from build123d import *
from OCP.BRepFilletAPI import BRepFilletAPI_MakeChamfer

# Parameters (mm, degrees)
SKETCH_2_W          = 8
SKETCH_2_H          = 200
EXTRUDE_1_DEPTH     = 10
SKETCH_3_W          = 2
SKETCH_3_H          = 30
EXTRUDE_2_DEPTH     = 10
SKETCH_4_R          = 1.65
CUT_EXTRUDE_1_DEPTH = 20
SKETCH_5_W          = 4
SKETCH_5_H          = 100
CUT_EXTRUDE_2_DEPTH = 20
CHAMFER_1_SIZE      = 5
CHAMFER_1_SIZE2     = 13.737387097
SKETCH_6_W          = 2
SKETCH_6_H          = 27.5
EXTRUDE_3_DEPTH     = 15
SKETCH_7_R          = 1.65
CUT_EXTRUDE_3_DEPTH = 10
SKETCH_8_R          = 1.6
CUT_EXTRUDE_4_DEPTH = 10


with BuildPart() as part:
    # 草图2 → 凸台-拉伸1 (new body)
    with BuildSketch(Plane(origin=(0, 0, 0), x_dir=(1, 0, 0), z_dir=(0, 1, 0))):
        Rectangle(SKETCH_2_W, SKETCH_2_H)
    extrude(amount=EXTRUDE_1_DEPTH)

    # 草图3 → 凸台-拉伸2 (add)
    with BuildSketch(Plane(origin=(0, 10, 0), x_dir=(1, 0, 0), z_dir=(0, 1, 0))):
        with Locations((-3, 0)):
            Rectangle(SKETCH_3_W, SKETCH_3_H)
        with Locations((3, 0)):
            Rectangle(SKETCH_3_W, SKETCH_3_H)
    extrude(amount=EXTRUDE_2_DEPTH)

    # 草图4 → 切除-拉伸1 (cut)
    with BuildSketch(Plane.ZY.offset(4)):
        with Locations((-7.5, 15)):
            Circle(SKETCH_4_R)
        with Locations((7.5, 15)):
            Circle(SKETCH_4_R)
    extrude(amount=-CUT_EXTRUDE_1_DEPTH, mode=Mode.SUBTRACT)

    # 草图5 → 切除-拉伸2 (cut)
    with BuildSketch(Plane(origin=(0, 10, 0), x_dir=(1, 0, 0), z_dir=(0, 1, 0))):
        Rectangle(SKETCH_5_W, SKETCH_5_H)
    extrude(amount=-CUT_EXTRUDE_2_DEPTH, mode=Mode.SUBTRACT)

    # 倒角1: one chamfer whose edges measure the first distance from different faces: ONE call of the kernel's chamfer builder (chamfer() names one face for all edges)
    chamfer_1_edges_1 = [part.edges().sort_by_distance(p)[0] for p in [
        (0, 0, 100),
    ]]
    chamfer_1_side_1 = [part.faces().sort_by_distance(p)[0] for p in [
        (0, 5, 100),
    ]]
    chamfer_1_edges_2 = [part.edges().sort_by_distance(p)[0] for p in [
        (0, 0, -100),
    ]]
    chamfer_1_side_2 = [part.faces().sort_by_distance(p)[0] for p in [
        (0, 5, -100),
    ]]
    chamfer_1 = BRepFilletAPI_MakeChamfer(part.part.solid().wrapped)
    for e in chamfer_1_edges_1:
        chamfer_1.Add(CHAMFER_1_SIZE, CHAMFER_1_SIZE2, e.wrapped, chamfer_1_side_1[0].wrapped)  # the first distance lies on this face
    for e in chamfer_1_edges_2:
        chamfer_1.Add(CHAMFER_1_SIZE, CHAMFER_1_SIZE2, e.wrapped, chamfer_1_side_2[0].wrapped)  # the first distance lies on this face
    add(Compound.cast(chamfer_1.Shape()), mode=Mode.REPLACE)

    # 草图6 → 凸台-拉伸3 (add)
    with BuildSketch(Plane(origin=(0, 10, 0), x_dir=(1, 0, 0), z_dir=(0, 1, 0))):
        with Locations((-3, 43.75)):
            Rectangle(SKETCH_6_W, SKETCH_6_H)
    extrude_3 = extrude(amount=EXTRUDE_3_DEPTH)

    # 镜向2: 凸台-拉伸3 across plane
    add(extrude_3.mirror(Plane.XY))

    # 草图7 → 切除-拉伸3 (cut)
    with BuildSketch(Plane.ZY.offset(4)):
        with Locations((80, 5)):
            Circle(SKETCH_7_R)
        with Locations((65, 5)):
            Circle(SKETCH_7_R)
        with Locations((-65, 5)):
            Circle(SKETCH_7_R)
        with Locations((-80, 5)):
            Circle(SKETCH_7_R)
    extrude(amount=-CUT_EXTRUDE_3_DEPTH, mode=Mode.SUBTRACT)

    # 草图8 → 切除-拉伸4 (cut)
    with BuildSketch(Plane(origin=(-2, 0, 0), x_dir=(0, 0, -1), z_dir=(1, 0, 0))):
        with Locations((-52.235249282, 21.351499314)):
            Circle(SKETCH_8_R)
        with Locations((-38.268733006, 15.880080566)):
            Circle(SKETCH_8_R)
        with Locations((38.268733006, 15.880080566)):
            Circle(SKETCH_8_R)
        with Locations((52.235249282, 21.351499314)):
            Circle(SKETCH_8_R)
    extrude(amount=-CUT_EXTRUDE_4_DEPTH, mode=Mode.SUBTRACT)


solid = part.part
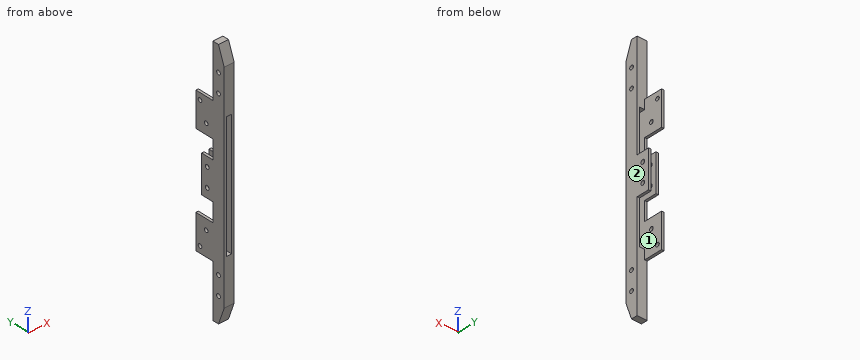
Verification items for the finished model (mm, model axes). Face numbers are marked on the shaded views. Give positions to 0.01 mm unless a question says otherwise; leave off trailing zeros. Write each loop counter-clockwise with the first axis right and the second up, starting at its lowest first coordinate (ties: lowest second). Pieces come first, ordered by that corner, then holes. Notation, with made-up numbers: (24.25, 1) -> (81.25, 1) arc R26 ccw to (81.25, 38) -> close; hole circle Ø10 at (2.25, 15.5). An arc over 180 degrees is marked (long way). Use CSV: the item, a comma, the result in double quotes.
(1) Release check for a two-part mould opening along Z. For the marked faces 1 and 2 record: +Z half, -Z half, draft (parallel to the pull), parting line (faces both ways), or undercut.
Derived:
face 1,"undercut"
face 2,"draft"
(2) Sectioned sample at C-C (z = 69.5). Record the cut outline in (x, y).
Derived:
outline,"(-4, 0) -> (4, 0) -> (4, 10) -> (-4, 10) -> close"
(3) Sectioned sample at B-B (z = -65). Record the cut outline in (x, y).
Derived:
outline,"(-4, 0) -> (4, 0) -> (4, 3.35) -> (-4, 3.35) -> close; (-4, 6.65) -> (4, 6.65) -> (4, 10) -> (-4, 10) -> close"
(4) Material ranges on L1, parallel to Z at x = -3.25, y = 11; L2, parallel to X at y = 15.25, z = 11.5; L3, parallel to Z at x = 1.5, y = 7.5, recorded low to high.
Derived:
L1,"z = -57.5 to -30, -15 to 15, 30 to 57.5"
L2,"x = -4 to -2, 2 to 4"
L3,"z = -100 to -50, 50 to 100"
(5) Go/stop test with flat-tipped pins: pin 1 (2.5 mm diameter, centred on y = 15, z = -7.5, fed in from +X); pin 2 (3.5 mm diameter, centred on y = 15.88, z = 38.27, fed in from +X); pin 3 (1 mm diameter, centred on x = -3, y = 21, fed in from -Z); pin 4 (2 mm diameter, centred on x = -3, y = 13.5, fed in from +Z). Record where each tip stops, or that it passes through.
Derived:
pin 1,"passes through"
pin 2,"stops at x = -2"
pin 3,"stops at z = -57.5"
pin 4,"stops at z = 57.5"
(6) Sectioned sample at A-A (z = 1.5). Record the cut outline in (x, y), plus the area to 3 significant figures.
Derived:
outline,"(-4, 0) -> (-2, 0) -> (-2, 20) -> (-4, 20) -> close; (2, 0) -> (4, 0) -> (4, 20) -> (2, 20) -> close"
area,"80.0 mm^2"
